Answer from the drawing. Dimensions are ordinates in mm from the lowest x, y and z of the part. A direction names the side the tool comes from. Round coordinates to 2 decimals unless told otherwise and drop trailing zeros. Loops run counter-clockwise (first coordinate to the right, second up) from the corner with the lowest first, then second, coordinate; pieces in that order, holes last. Notation, with made-up numbers: M 54.25,-1.75 L 68.25,-1.75 A20 ccw 68.25,23.25 Z; hole C 33,44 d5. An arc over 180 degrees is marked long. Answer as a JSON object with one key per item and string values.
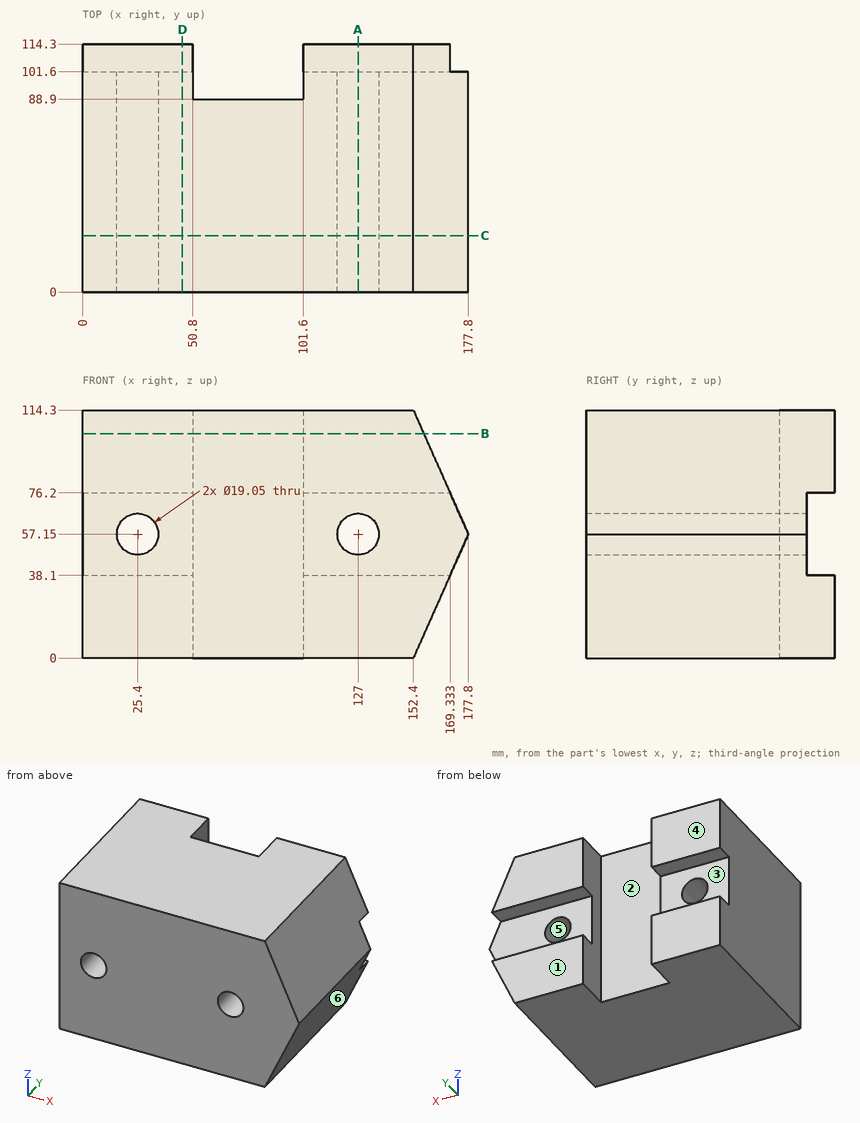
Item 1: Which of the six approach directions +Z, -Z, +X, -X, +Y, -Y give full straight-line access (tool end or side, diameter ignored) to the marked faces 1, 2 and 3?
Values follow:
{"face 1": "+Z, -Z, +X, -X, +Y", "face 2": "+Z, -Z, +Y", "face 3": "+X, -X, +Y"}
Item 2: The part is cut by section B-B (z = 103.5). Give the vertices of the cut face in (x, y), then the cut area to 3 significant figures.
Values follow:
{"outline": "M 0,0 L 157.2,0 L 157.2,114.3 L 101.6,114.3 L 101.6,88.9 L 50.8,88.9 L 50.8,114.3 L 0,114.3 Z", "area": "16,700 mm^2"}
Item 3: The part is cut by section C-C (y = 26). Give the number of separate pieces and of enclosed holes in the cut face, then the cut area to 3 significant figures.
Values follow:
{"separate pieces": "1", "enclosed holes": "2", "area": "18,300 mm^2"}
Item 4: Determine the mould class of the marked faces 4, 5 and 6 for opening direction X: released by +X, released by -X, zero draft, split by the parting line, or undercut.
Values follow:
{"face 4": "zero draft", "face 5": "undercut", "face 6": "released by +X"}
Item 5: Straight lines are drawn through the part: line 1 (X direction, y = 81, z = 57.15) (1 decimal); line 2 (Z direction, x = 127, y = 77) (1 decimal); line 3 (X direction, y = 18, z = 64.5) (1 decimal). For each, find the intervals that lie inside material, in ascending order.
Values follow:
{"line 1": "0 to 15.9, 34.9 to 117.5, 136.5 to 177.8", "line 2": "0 to 47.6, 66.7 to 114.3", "line 3": "0 to 19.3, 31.5 to 120.9, 133.1 to 174.5"}
Item 6: Flat-ended cylindrical pins translate along their axes: P1, Ø22, axis at x = 127, z = 57.15, coming from the +Y side; P2, Ø1, axis at y = 70, z = 100, coming from the +X side; P3, Ø2, axis at x = 71, z = 33, coming from the +Y side. Find the tip coordinate at first contact, or state that the pin passes through.
Values follow:
{"P1": "y = 101.6", "P2": "x = 158.98", "P3": "y = 88.9"}
Item 7: The part is cut by section A-A (x = 127). Give the vertices of the cut face in (y, z) (1 decimal), then the cut area to 3 significant figures.
Values follow:
{"outline": "M 0,0 L 114.3,0 L 114.3,38.1 L 101.6,38.1 L 101.6,47.6 L 0,47.6 Z; M 0,66.7 L 101.6,66.7 L 101.6,76.2 L 114.3,76.2 L 114.3,114.3 L 0,114.3 Z", "area": "10,600 mm^2"}
Item 8: The part is cut by section D-D (x = 46). Give the vertices of the cut face in (y, z), then the cut area to 3 significant figures.
Values follow:
{"outline": "M 0,0 L 114.3,0 L 114.3,38.1 L 101.6,38.1 L 101.6,76.2 L 114.3,76.2 L 114.3,114.3 L 0,114.3 Z", "area": "12,600 mm^2"}
